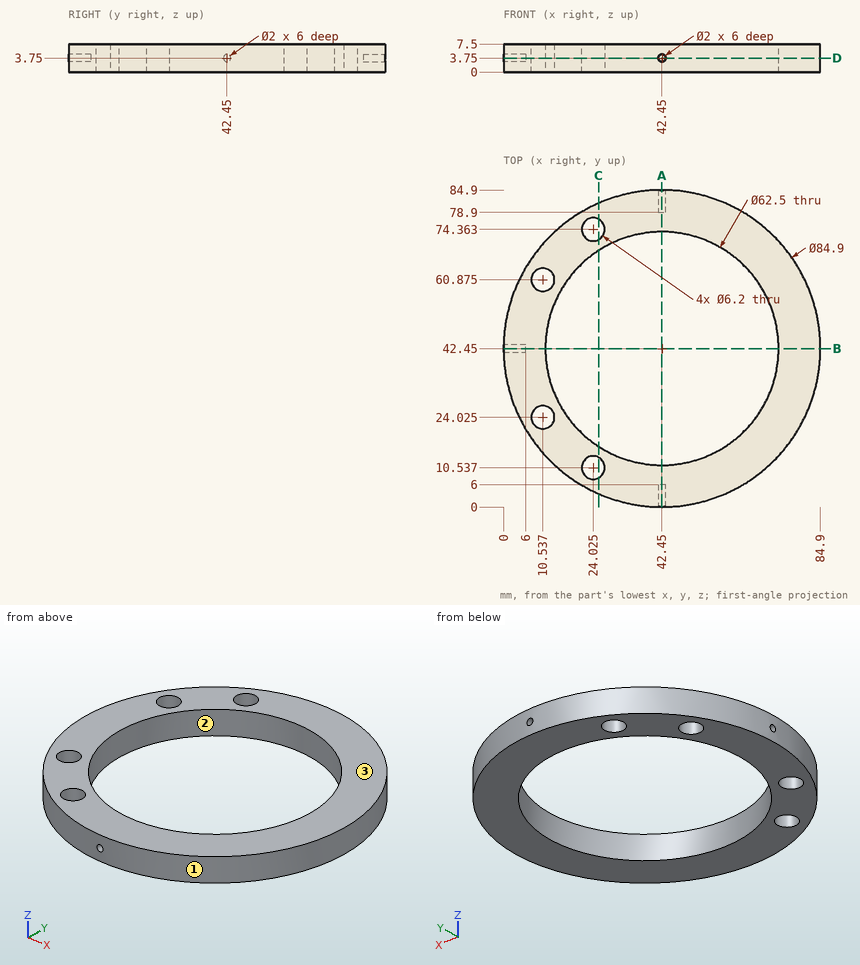
Geometry: see drawing. Coordinates: mm, zero at the bounding-box minimum. Coordinates: 2 decimals unless noted, no trailing zeros. Write each loop counter-clockwise with the first axis right and the second up, starting at its lowest first coordinate (ties: lowest second). Pieces come first, ordered by that corner, then holes. Notation, with made-up numbers: (3.5, 51) - (26.5, 51) arc R15 ccw to (26.5, 72) - close; hole circle Ø11 at (87.25, -10). An arc over 180 degrees is marked (long way). Put each result on its own line as item: value. Start each with the question number.
1) Cut plane B-B (y = 42.45). Return the cut outline in (x, z), plus the area to 3 significant figures.
2) Contact query for flat-ended pins moving along their axis: pin 1 (5.5 mm diameter, centred on x = 10.54, y = 60.88, fed in from +Z); pin 2 (3 mm diameter, centred on x = 55, z = 1, fed in from -Y); pin 3 (0.6 mm diameter, centred on y = 42.5, z = 4, fed in from -X); pin 4 (1 mm diameter, centred on x = 42.5, z = 3.5, fed in from +Y). Output: stop coordinate, or through.
3) Cut plane C-C (x = 25.5). Return the cut outline in (y, z), plus the area to 3 significant figures.
4) Cut plane D-D (z = 3.75). Return the cut outline in (x, y) (3 decimals), plus the area to 3 significant figures.
5) Cut plane A-A (x = 42.45). Return the cut outline in (y, z), plus the area to 3 significant figures.
6) Ray query, L1, parallel to Y at x = 10.5, z = 4 (3 decimals); L2, parallel to Z at x = 42.45, y = 3.5; L3, parallel to Y at x = 8, z = 1.25. Return the intervals inside material, ascending.
7) Mould query, pull axis Y, two halves, no side actions, for the marked faces 1, 2 and 3. Classes: pulls with the +Y half, pulls with the -Y half, needs draft (parallel to the pull), parting line crosses it, or undercut.
Resolved:
1. outline: (0, 0) - (11.2, 0) - (11.2, 7.5) - (0, 7.5) - (0, 4.75) - (6, 4.75) - (6, 2.75) - (0, 2.75) - close; (73.7, 0) - (84.9, 0) - (84.9, 7.5) - (73.7, 7.5) - close
1. area: 156 mm2
2. pin 1: passes through
2. pin 2: stops at y = 1.46
2. pin 3: stops at x = 6
2. pin 4: stops at y = 78.9
3. outline: (3.53, 0) - (7.81, 0) - (7.81, 7.5) - (3.53, 7.5) - close; (13.26, 0) - (16.2, 0) - (16.2, 7.5) - (13.26, 7.5) - close; (68.7, 0) - (71.64, 0) - (71.64, 7.5) - (68.7, 7.5) - close; (77.09, 0) - (81.37, 0) - (81.37, 7.5) - (77.09, 7.5) - close
3. area: 108 mm2
4. outline: (0.012, 41.45) arc R42.45 ccw to (41.45, 0.012) - (41.45, 6) - (43.45, 6) - (43.45, 0.012) arc R42.45 ccw to (43.45, 84.888) - (43.45, 78.9) - (41.45, 78.9) - (41.45, 84.888) arc R42.45 ccw to (0.012, 43.45) - (6, 43.45) - (6, 41.45) - close; hole circle Ø6.2 at (10.537, 24.025); hole circle Ø6.2 at (10.537, 60.875); hole circle Ø62.5 at (42.45, 42.45); hole circle Ø6.2 at (24.025, 10.537); hole circle Ø6.2 at (24.025, 74.363)
4. area: 2,440 mm2
5. outline: (0, 0) - (11.2, 0) - (11.2, 7.5) - (0, 7.5) - (0, 4.75) - (6, 4.75) - (6, 2.75) - (0, 2.75) - close; (73.7, 0) - (84.9, 0) - (84.9, 2.75) - (78.9, 2.75) - (78.9, 4.75) - (84.9, 4.75) - (84.9, 7.5) - (73.7, 7.5) - close
5. area: 144 mm2
6. L1: y = 14.5 to 20.925, 27.125 to 57.775, 63.975 to 70.4
6. L2: z = 0 to 2.75, 4.75 to 7.5
6. L3: y = 17.65 to 22.24, 25.81 to 59.09, 62.66 to 67.25
7. face 1: parting line crosses it
7. face 2: undercut
7. face 3: needs draft
